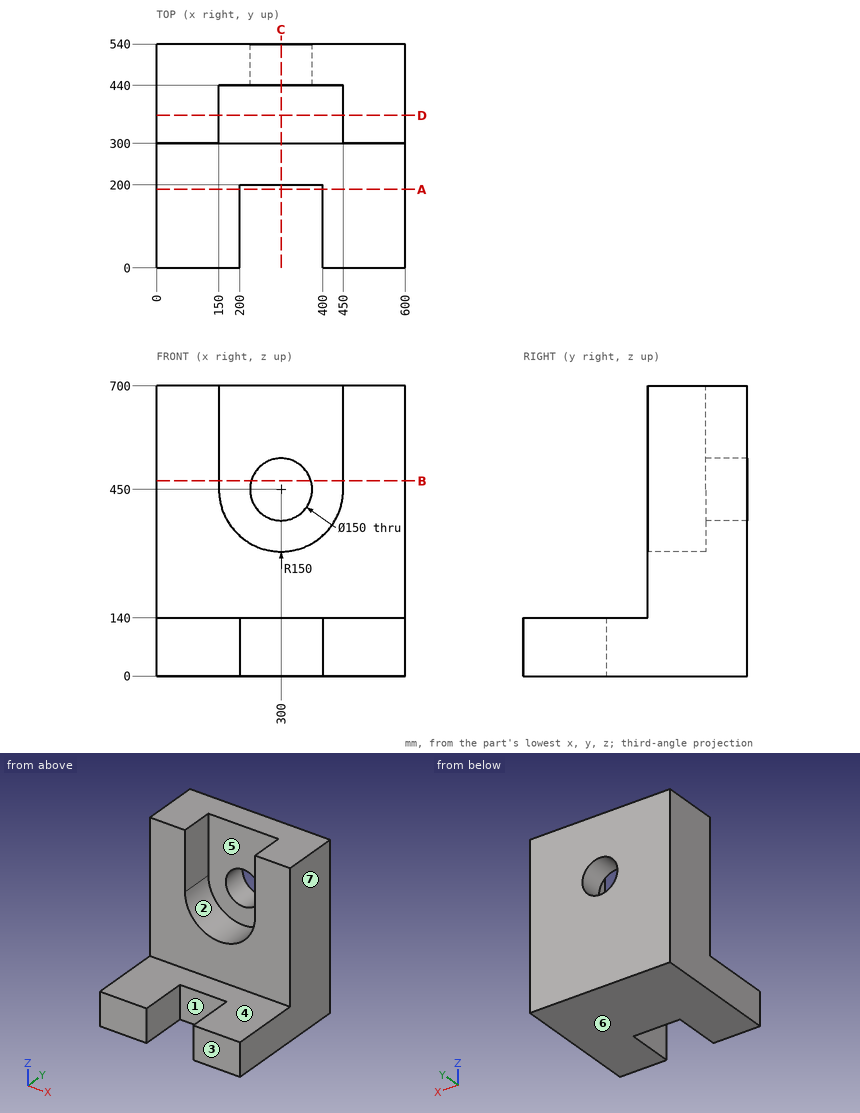
Check sheet for the drawn part. Datum: minimum x, y, z corner. Units: mm. A direction names the side the tool comes from. Give positions to 0.01 mm unless a question says otherwise; leave off trailing zeros. Order: outer loops, then holes, each group sorted by start corner. A loop starts at its lowest first (then second) coordinate and runs counter-clockwise, first axis right, second up. Notation, with made-up numbers: (47, 43.25) -> (54, 43.25) arc R17 cw to (54, 53.25) -> close; hole circle Ø2 at (-28.75, 64). An arc over 180 degrees is marked (long way). Answer as CSV lines item,"result".
Q1. Sectioned sample at C-C on x = 300. Record the cut outline in (y, z).
Solutions:
outline,"(200, 0) -> (540, 0) -> (540, 375) -> (440, 375) -> (440, 300) -> (300, 300) -> (300, 140) -> (200, 140) -> close; (440, 525) -> (540, 525) -> (540, 700) -> (440, 700) -> close"
Q2. Release check for a two-part mould opening along X. For the marked faces 5, 6 and 7 record: +X half, -X half, draft (parallel to the pull), parting line (faces both ways), or undercut.
Solutions:
face 5,"undercut"
face 6,"draft"
face 7,"+X half"
Q3. Access from +Z, -Z, +X, -X, +Y, -Y to the whole of each face (thin tool, end or side, straight path). Record for the marked faces 1, 2, 3 and 4.
Solutions:
face 1,"+Z, -Z, -Y"
face 2,"+Z, -Y"
face 3,"+Z, -Z, +X, -X, -Y"
face 4,"+Z, +X, -X, -Y"
Q4. Depth check by flat-ended pin: pin 1 (3 mm diameter, centred on x = 504.5, z = 558, fed in from -Y). Enter the tip coordinate at first touch or a pass-through.
Solutions:
pin 1,"stops at y = 300"
Q5. Sectioned sample at D-D on y = 368. Record the cut outline in (x, z), plus the area to 3 significant figures.
Solutions:
outline,"(0, 0) -> (600, 0) -> (600, 700) -> (450, 700) -> (450, 450) arc R150 cw to (150, 450) -> (150, 700) -> (0, 700) -> close"
area,"310,000 mm²"
Q6. Sectioned sample at B-B on z = 471. Record the cut outline in (x, y).
Solutions:
outline,"(0, 300) -> (150, 300) -> (150, 440) -> (228, 440) -> (228, 540) -> (0, 540) -> close; (372, 440) -> (450, 440) -> (450, 300) -> (600, 300) -> (600, 540) -> (372, 540) -> close"
Q7. Sectioned sample at A-A on y = 189.5. Record the cut outline in (x, z), plus the area to 3 significant figures.
Solutions:
outline,"(0, 0) -> (200, 0) -> (200, 140) -> (0, 140) -> close; (400, 0) -> (600, 0) -> (600, 140) -> (400, 140) -> close"
area,"56,000 mm²"
Q8. Scan lines: probe 1 along Z at (x, y) = (300, 470); probe 2 along X at (y, z) = (154, 38); probe 3 along Y at (x, z) = (26, 658). Record each from-to range of solid material in increasing order.
Solutions:
probe 1,"z = 0 to 375, 525 to 700"
probe 2,"x = 0 to 200, 400 to 600"
probe 3,"y = 300 to 540"
